from build123d import *

# Parameters (mm, degrees)
F0_R     = 3.1
F1_DEPTH = 3.175


with BuildPart() as f1:
    # F0 (on Front) → F1 (new body)
    with BuildSketch(Plane.XZ):
        with BuildLine():
            ThreePointArc((-88.9, 0), (-92, 3.1), (-95.1, 0))
            ThreePointArc((-95.1, 0), (-92, -3.1), (-88.9, 0))
        make_face()
        with Locations((92, 0)):
            Circle(F0_R)
        with BuildLine():
            ThreePointArc((100, 0), (97.071068, 7.071068), (90, 10))
            Line((90, 10), (-90, 10))
            ThreePointArc((-90, 10), (-97.071068, 7.071068), (-100, 0))
            ThreePointArc((-100, 0), (-97.071068, -7.071068), (-90, -10))
            Line((-90, -10), (90, -10))
            ThreePointArc((90, -10), (97.071068, -7.071068), (100, 0))
        make_face()
        with BuildLine():
            ThreePointArc((-88.9, 0), (-92, -3.1), (-95.1, 0))
            ThreePointArc((-95.1, 0), (-92, 3.1), (-88.9, 0))
        make_face(mode=Mode.SUBTRACT)
        with Locations((92, 0)):
            Circle(F0_R, mode=Mode.SUBTRACT)
    extrude(amount=F1_DEPTH)


solid = f1.part
Source: CAD feature listing. Evaluate the final solid. Frame: model axes, mm. Round coordinates to 2 decimals unless told otherwise and drop trailing zeros. Write each loop counter-clockwise with the first axis right and the second up, starting at its lowest first coordinate (ties: lowest second). Pieces come first, ordered by that corner, then holes. Notation, with made-up numbers: M 18,75 L 29,75 A20 ccw 29,107 Z; hole C -19.5,-4.75 d4. An arc over 180 degrees is marked long. One line per item, written item: value. Start each with the question number.
Item 1: Section query B-B (x = 92). Return the cut outline in (y, z) (3 decimals).
Item 2: Pin query (flat end, axial travel): pin 1 (1.5 mm diameter, centred on x = 11, z = 6, fed in from +Y); pin 2 (3.5 mm diameter, centred on x = -92, z = 0, fed in from -Y). Return the tip coordinate at first contact, or that it passes through.
Item 3: Section query A-A (y = -0.6). Return the cut outline in (x, z), plus the area to 3 significant figures.
Item 4: Ray query, L1, parallel to X at y = -2.95, z = -0.5; L2, parallel to X at y = -2.75, z = 1; L3, parallel to Z at x = -92, y = -0.85. Return the intervals inside material, ascending. Write a range as from..to.
Item 5: Mould query, pull axis Z, two halves, no side actions, for faces 1 (the flat face through (-1, 0, 0)), 2 (the cylindrical face through (94.957, -1.565, 0.931)), 3 (the flat face through (1, -2, 10)). Classes: pulls with the +Z half, pulls with the -Z half, needs draft (parallel to the pull), parting line crosses it, or undercut.
Result set:
1. outline: M -3.175,-9.798 L 0,-9.798 L 0,-3.1 L -3.175,-3.1 Z; M -3.175,3.1 L 0,3.1 L 0,9.798 L -3.175,9.798 Z
2. pin 1: stops at y = 0
2. pin 2: passes through
3. outline: M -100,0 A10 ccw -90,-10 L 90,-10 A10 ccw 100,0 A10 ccw 90,10 L -90,10 A10 ccw Z; hole C -92,0 d6.2; hole C 92,0 d6.2
3. area: 3,850 mm²
4. L1: x = -99.99..-95.06, -88.94..88.94, 95.06..99.99
4. L2: x = -99.95..-94.93, -89.07..89.07, 94.93..99.95
4. L3: z = -9.8..-3.1, 3.1..9.8
5. face 1: needs draft
5. face 2: undercut
5. face 3: pulls with the +Z half
